```python
from build123d import *

# Parameters (mm, degrees)
SKETCH1_R           = 3.550069734
SKETCH1_W           = 5.542666669
SKETCH1_H           = 3.000080526
BOSS_EXTRUDE1_DEPTH = 3.175


with BuildPart() as part:
    # Sketch1 → Boss-Extrude1 (new body)
    with BuildSketch(Plane(origin=(0, 0, 0), x_dir=(1, 0, 0), z_dir=(0, 1, 0))):
        Polygon((21.594595228, 0.978080338), (21.594595228, -2.022000189), (24.059548337, -2.022000189), (24.059548337, -21.222556575), (22.761975246, -21.222556575), (22.761975246, -24.222705465), (12.779622417, -24.222705465), (12.779622417, -21.222556575), (-7.185015001, -21.222556575), (-7.185015001, -24.222705465), (-22.158349273, -24.222705465), (-22.158349273, -21.222556575), (-23.456117337, -21.222556575), (-23.456117337, -2.021873227), (-13.573249368, -2.021873227), (-13.573249368, 0.978275664), (-23.456117336, 0.978275664), (-23.456117336, 24.479227112), (-22.158349272, 24.479227112), (-22.158349272, 27.47917091), (-17.167172857, 27.47917091), (-17.167172857, 24.479227112), (-14.172644433, 24.479227112), (-14.172644433, 27.47917091), (-9.181477767, 27.47917091), (-9.181477767, 24.479227112), (9.784899021, 24.479227112), (9.784899021, 27.47917091), (22.761975247, 27.47917091), (22.761975247, 24.479227112), (24.059548338, 24.479227112), (24.08510927, 24.47910015), (24.08510927, 7.98726625), (27.405593185, 7.98726625), (27.405593185, 4.687262638), (24.08510927, 4.687262638), (24.08510927, 0.978080338), align=None)
        with Locations(Location((0.24664544, 1.581901392, 0), (0, 0, 270))):
            Circle(SKETCH1_R, mode=Mode.SUBTRACT)
        with Locations((17.647010615, -0.521959927)):
            Rectangle(SKETCH1_W, SKETCH1_H, mode=Mode.SUBTRACT)
        with BuildLine():
            Line((-0.638404245, 11.51973711), (-0.638404245, 16.519887597))
            ThreePointArc((-0.638404245, 16.519887597), (0.259966955, 17.418258798), (1.158338156, 16.519887597))
            Line((1.158338156, 16.519887597), (1.158338156, 11.51973711))
            ThreePointArc((1.158338156, 11.51973711), (0.259966955, 10.62136591), (-0.638404245, 11.51973711))
        make_face(mode=Mode.SUBTRACT)
        with BuildLine():
            Line((-0.651633149, -13.218614368), (-0.651633149, -8.218395516))
            ThreePointArc((-0.651633149, -8.218395516), (0.246738051, -7.320024316), (1.145109252, -8.218395516))
            Line((1.145109252, -8.218395516), (1.145109252, -13.218614368))
            ThreePointArc((1.145109252, -13.218614368), (0.246738051, -14.116985568), (-0.651633149, -13.218614368))
        make_face(mode=Mode.SUBTRACT)
    extrude(amount=BOSS_EXTRUDE1_DEPTH)


solid = part.part
```
Model file for the job. Use its own axes, mm. A direction names the side the tool comes from. Coordinates: 2 decimals unless noted, no trailing zeros. Order: outer loops, then holes, each group sorted by start corner. A loop starts at its lowest first (then second) coordinate and runs counter-clockwise, first axis right, second up. Notation, with made-up numbers: (40.25, 55) -> (76.25, 55) arc R19 cw to (76.25, 82) -> close; hole circle Ø7 at (37.5, -35). An arc over 180 degrees is marked (long way). Return JSON: item names as keys, results as strings.
Item 1: Slice it at D-D (y = 2.2). Count the separate pieces of the cut face and the enclosed holes in it, then the cut area to 3 significant figures.
Model answer:
{"separate pieces": "1", "enclosed holes": "4", "area": "2,210 mm²"}
Item 2: Pin check, flat tips, straight feed: P1, Ø0.9, axis at y = 1.5, z = 23, coming from the +X side; P2, Ø1, axis at y = 2, z = -20, coming from the +X side; P3, Ø0.9, axis at y = 1.5, z = 23, coming from the -X side. Stop position of each tip, or through.
Model answer:
{"P1": "stops at x = 22.76", "P2": "stops at x = 24.09", "P3": "stops at x = -22.16"}
Item 3: Slice it at C-C (z = -22). Write the cut outline in (x, y) (3 decimals).
Model answer:
{"outline": "(-23.456, 0) -> (24.085, 0) -> (24.085, 3.175) -> (-23.456, 3.175) -> close"}
Item 4: 3-axis set-ups, long thin cutter, end or side, ignore diameter. For faces 1 (the face through (18, 2, -0.978)), 2 (the face through (-18, 2, -0.978)), 3 (the face through (24.06, 2, 11)), 4 (the face through (-22.158, 2, 23)): which of +Z, -Z, +X, -X, +Y, -Y reach the whole face in a straight line?
Model answer:
{"face 1": "+Y, -Y", "face 2": "-X, +Y, -Y", "face 3": "+Z, +X, +Y, -Y", "face 4": "+Z, -X, +Y, -Y"}
Item 5: Mould opens along Z. For faces 5 (the face through (-0.638, 2, -14)), 6 (the face through (2, 0, 4)), 7 (the face through (-0.652, 2, 11)), 8 (the face through (23, 2, -24.479)) say: pulls with the +Z half, pulls with the -Z half, needs draft (parallel to the pull), parting line crosses it, or undercut.
Model answer:
{"face 5": "undercut", "face 6": "needs draft", "face 7": "undercut", "face 8": "pulls with the -Z half"}
Item 6: Wall check: line 1 along X through (y, z) = (1.8, -14); line 2 along Z through (x, y) = (-15, 1.2); line 3 along X through (y, z) = (0.55, -8.5). Give the ranges that are in metal, low to high. Write a range as from..to.
Model answer:
{"line 1": "x = -23.46..-0.64, 1.16..24.09", "line 2": "z = -24.48..-0.98, 2.02..24.22", "line 3": "x = -23.46..24.09"}
Item 7: Slice it at B-B (x = -18.5). Write the cut outline in (y, z) (3 decimals).
Model answer:
{"outline": "(0, -27.479) -> (3.175, -27.479) -> (3.175, -0.978) -> (0, -0.978) -> close; (0, 2.022) -> (3.175, 2.022) -> (3.175, 24.223) -> (0, 24.223) -> close"}
Item 8: Slice it at A-A (z = 9). Write the cut outline in (x, y) (3 decimals), then the cut area to 3 significant figures.
Model answer:
{"outline": "(-23.456, 0) -> (-0.652, 0) -> (-0.652, 3.175) -> (-23.456, 3.175) -> close; (1.145, 0) -> (24.06, 0) -> (24.06, 3.175) -> (1.145, 3.175) -> close", "area": "145 mm²"}
